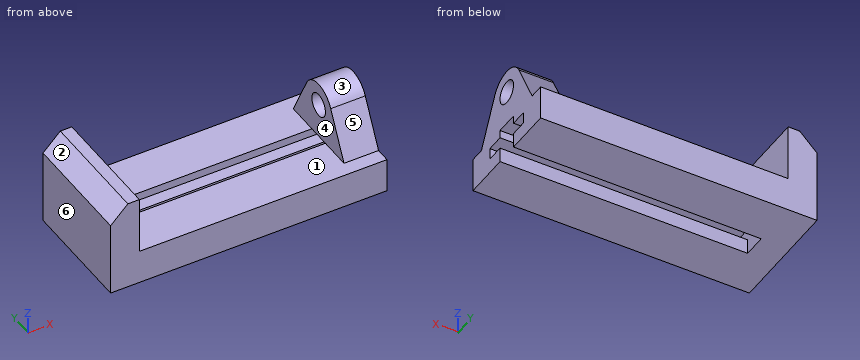
from build123d import *

# Parameters (mm, degrees)
F1_DEPTH = 127
F3_DEPTH = 234.95
F4_R     = 12.7
F5_DEPTH = 38.1


with BuildPart() as f1:
    # F0 (on Front) → F1 (new body)
    with BuildSketch(Plane.XZ):
        Polygon((0, 82.55), (0, 0), (31.75, 0), (31.75, 101.6), (19.05, 101.6), align=None)
    extrude(amount=F1_DEPTH)

    # F2 (on face) → F3 (join)
    with BuildSketch(Plane.YZ.offset(31.75)):
        Polygon((-127, 38.1), (-127, 0), (-76.2, 0), (-76.2, 16.51), (-95.25, 16.51), (-95.25, 29.21), (-76.2, 29.21), (-76.2, 38.1), align=None)
        Polygon((-50.8, 16.51), (-50.8, 0), (0, 0), (0, 38.1), (-50.8, 38.1), (-50.8, 29.21), (-31.75, 29.21), (-31.75, 16.51), align=None)
    extrude(amount=F3_DEPTH)

    # F4 (on face) → F5 (join)
    with BuildSketch(Plane.YZ.offset(266.7)):
        with BuildLine():
            Line((-127, 38.1), (-127, 0))
            Line((-127, 0), (-76.2, 0))
            Line((-76.2, 0), (-76.2, 16.51))
            Line((-76.2, 16.51), (-95.25, 16.51))
            Line((-95.25, 16.51), (-95.25, 29.21))
            Line((-95.25, 29.21), (-76.2, 29.21))
            Line((-76.2, 29.21), (-76.2, 38.1))
            Line((-76.2, 38.1), (-50.8, 38.1))
            Line((-50.8, 38.1), (-50.8, 29.21))
            Line((-50.8, 29.21), (-31.75, 29.21))
            Line((-31.75, 29.21), (-31.75, 16.51))
            Line((-31.75, 16.51), (-50.8, 16.51))
            Line((-50.8, 16.51), (-50.8, 0))
            Line((-50.8, 0), (0, 0))
            Line((0, 0), (0, 38.1))
            Line((0, 38.1), (-15.875, 38.1))
            Line((-15.875, 38.1), (-40.814084, 87.624062))
            ThreePointArc((-40.814084, 87.624062), (-63.5, 101.6), (-86.185916, 87.624062))
            Line((-86.185916, 87.624062), (-111.125, 38.1))
            Line((-111.125, 38.1), (-127, 38.1))
        make_face()
        with Locations((-63.5, 76.2)):
            Circle(F4_R, mode=Mode.SUBTRACT)
    extrude(amount=F5_DEPTH)


solid = f1.part
Build history of the part. All positions in model axes, mm. Face numbers are marked on the shaded views. A direction names the side the tool comes from. Coordinates: 2 decimals unless noted, no trailing zeros. Order: outer loops, then holes, each group sorted by start corner. A loop starts at its lowest first (then second) coordinate and runs counter-clockwise, first axis right, second up. Notation, with made-up numbers: (-15, -30.75) - (43, -30.75) arc R17 ccw to (43, -15.75) - close; hole circle Ø6 at (20.25, 53). An arc over 180 degrees is marked (long way). Write item = value, one per line. Start each with the question number.
1) Two-plate mould, pull along X, no slides. Class the marked faces 1, 2 and 3: pulls with the +X half, pulls with the -X half, needs draft (parallel to the pull), parting line crosses it, or undercut.
2) Saw through at D-D on z = 12. Write the cut outline in (x, y), then the cut area to 3 significant figures.
3) Saw through at A-A on x = 209. Write the cut outline in (y, z).
4) Wall check: line 1 along Y through (x, z) = (38.5, 6); line 2 along Z through (x, y) = (280, -63); line 3 along X through (y, z) = (-54.5, 62.5). Give the ranges that are in metal, low to high. Write a range as from..to.
5) Saw through at C-C on z = 76.2. Write the cut outline in (x, y).
6) Flat gauge pins, fed straight in: pin 1 Ø12.5 at (x, y) = (287.5, -61) entering from -Z; pin 2 Ø3 at (x, y) = (129.5, -75.5) entering from +Z. Where does each tip first touch, or does it go through?
7) Saw through at B-B on y = -63.5. Write the cut outline in (x, z).
8) 3-axis set-ups, long thin cutter, end or side, ignore diameter. For the marked faces 4, 5 and 6: which of +Z, -Z, +X, -X, +Y, -Y reach the whole face in a straight line?
From the geometry:
q1.face_1 = undercut
q1.face_2 = pulls with the -X half
q1.face_3 = needs draft
q2.outline = (0, -127) - (304.8, -127) - (304.8, -76.2) - (31.75, -76.2) - (31.75, -50.8) - (304.8, -50.8) - (304.8, 0) - (0, 0) - close
q2.area = 31,800 mm^2
q3.outline = (-127, 0) - (-76.2, 0) - (-76.2, 16.51) - (-95.25, 16.51) - (-95.25, 29.21) - (-76.2, 29.21) - (-76.2, 38.1) - (-127, 38.1) - close; (-50.8, 0) - (0, 0) - (0, 38.1) - (-50.8, 38.1) - (-50.8, 29.21) - (-31.75, 29.21) - (-31.75, 16.51) - (-50.8, 16.51) - close
q4.line_1 = -127..-76.2, -50.8..0
q4.line_2 = 38.1..63.51, 88.89..101.6
q4.line_3 = 0..31.75, 266.7..304.8
q5.outline = (0, -127) - (31.75, -127) - (31.75, 0) - (0, 0) - close; (266.7, -91.94) - (304.8, -91.94) - (304.8, -76.2) - (266.7, -76.2) - close; (266.7, -50.8) - (304.8, -50.8) - (304.8, -35.06) - (266.7, -35.06) - close
q6.pin_1 = 38.1
q6.pin_2 = 38.1
q7.outline = (0, 0) - (31.75, 0) - (31.75, 101.6) - (19.05, 101.6) - (0, 82.55) - close; (266.7, 38.1) - (304.8, 38.1) - (304.8, 63.5) - (266.7, 63.5) - close; (266.7, 88.9) - (304.8, 88.9) - (304.8, 101.6) - (266.7, 101.6) - close
q8.face_4 = +Z, +Y, -Y
q8.face_5 = +Z, +X, -Y
q8.face_6 = +Z, -Z, -X, +Y, -Y
